```python
from build123d import *

# Parameters (mm, degrees)
SKETCH1_W                                         = 19.05
SKETCH1_H                                         = 19.05
BOSS_EXTRUDE1_DEPTH                               = 6.35
SKETCH2_W                                         = 6.444113488
SKETCH2_H                                         = 19.05
BOSS_EXTRUDE2_DEPTH                               = 12.7
CSK_FOR_8_FLAT_HEAD_MACHINE_SCREW_100_D           = 4.9149
CSK_FOR_8_FLAT_HEAD_MACHINE_SCREW_100_DEPTH       = 23.368
CSK_FOR_8_FLAT_HEAD_MACHINE_SCREW_100_CSINK_D     = 8.4328
CSK_FOR_8_FLAT_HEAD_MACHINE_SCREW_100_CSINK_ANGLE = 100
CSK_FOR_8_FLAT_HEAD_MACHINE_SCREW_100_TIP         = 1.476584928
SKETCH5_R                                         = 1.5875
CUT_EXTRUDE1_DEPTH                                = 12.7
FILLET1_R                                         = 2.54
FILLET2_R                                         = 7.62


with BuildPart() as part:
    # Sketch1 → Boss-Extrude1 (new body)
    with BuildSketch(Plane(origin=(0, 0, 0), x_dir=(1, 0, 0), z_dir=(0, 1, 0))):
        with Locations((9.525, 9.525)):
            Rectangle(SKETCH1_W, SKETCH1_H)
    extrude(amount=BOSS_EXTRUDE1_DEPTH)

    # Sketch2 → Boss-Extrude2 (add)
    with BuildSketch(Plane(origin=(0, 6.35, 0), x_dir=(1, 0, 0), z_dir=(0, 1, 0))):
        with Locations((3.222056744, 9.525)):
            Rectangle(SKETCH2_W, SKETCH2_H)
    extrude(amount=BOSS_EXTRUDE2_DEPTH)

    # CSK for #8 Flat Head Machine Screw (100)1
    with Locations(Plane(origin=(0, 6.35, 0), x_dir=(1, 0, 0), z_dir=(0, 1, 0))):
        with Locations((12.7, 13.97), (12.7, 5.08)):
            CounterSinkHole(CSK_FOR_8_FLAT_HEAD_MACHINE_SCREW_100_D / 2, CSK_FOR_8_FLAT_HEAD_MACHINE_SCREW_100_CSINK_D / 2, depth=CSK_FOR_8_FLAT_HEAD_MACHINE_SCREW_100_DEPTH, counter_sink_angle=CSK_FOR_8_FLAT_HEAD_MACHINE_SCREW_100_CSINK_ANGLE)
            with Locations((0, 0, -(CSK_FOR_8_FLAT_HEAD_MACHINE_SCREW_100_DEPTH + CSK_FOR_8_FLAT_HEAD_MACHINE_SCREW_100_TIP / 2))):  # 118° drill point
                Cone(0, CSK_FOR_8_FLAT_HEAD_MACHINE_SCREW_100_D / 2, CSK_FOR_8_FLAT_HEAD_MACHINE_SCREW_100_TIP, mode=Mode.SUBTRACT)

    # Sketch5 → Cut-Extrude1 (cut)
    with BuildSketch(Plane(origin=(6.444113488, 0, 0), x_dir=(0, 0, -1), z_dir=(1, 0, 0))):
        with Locations((9.525, 12.7)):
            Circle(SKETCH5_R)
    extrude(amount=-CUT_EXTRUDE1_DEPTH, mode=Mode.SUBTRACT)

    # Fillet1
    fillet1_edges = [part.edges().sort_by_distance(p)[0] for p in [
        (6.444113488, 6.35, -9.525),
    ]]
    fillet(fillet1_edges, radius=FILLET1_R)

    # Fillet2
    fillet2_edges = [part.edges().sort_by_distance(p)[0] for p in [
        (0, 0, -9.525),
    ]]
    fillet(fillet2_edges, radius=FILLET2_R)


solid = part.part
```
The model under review builds one solid part; all positions refer to its coordinate system, in mm. A direction names the side the tool comes from. Round coordinates to 2 decimals unless told otherwise and drop trailing zeros. Order: outer loops, then holes, each group sorted by start corner. A loop starts at its lowest first (then second) coordinate and runs counter-clockwise, first axis right, second up. Notation, with made-up numbers: (56, -10.5) -> (67, -10.5) arc R22 ccw to (67, 5.5) -> close; hole circle Ø8 at (36, 27). An arc over 180 degrees is marked (long way). One line per item, written item: value. Start each with the question number.
Q1. Take a section at B-B (x = 12.7). Write out the cut boundary in (y, z).
Q2. Take a section at D-D (y = 17.5). Write out the cut boundary in (x, z).
Q3. Mouldability with a two-part tool opening along Z and no side actions: class faces 3 (the face through (19.05, 3, -9)), 4 (the face through (14.65, 2.403, -3.585)), 5 (the face through (5, 7, -19.05)) as released by +Z, released by -Z, zero draft, split by the parting line, or undercut.
Q4. Wall thickness on line 1 (Z direction, x = 12.7, y = 3.55); line 2 (Y direction, x = 13, z = -9.5); line 3 (X direction, y = 16, z = -14.5): over which ranges is each line inside the solid? List them lowest first.
Q5. Machinability: for faces 1 (the face through (13, 0, -10)), 2 (the face through (6.444, 15, -9)), which of the approach directions +Z, -Z, +X, -X, +Y, -Y give a long, thin tool a straight path to every point of the face, cutting with its end or side? Answer none if there is none.
Q6. Take a section at A-A (y = 12.7). Write out the cut boundary in (x, z).
Q7. Clearance check with flat-ended pins moving along their axes: pin 1 Ø1.5 at (y, z) = (13, -3) entering from +X; pin 2 Ø5 at (x, z) = (13.5, -7) entering from +Y. State where each tip first meets the part, or that it passes through.
Reported:
1. outline: (0, -19.05) -> (6.35, -19.05) -> (6.35, -18.19) -> (4.87, -16.43) -> (0, -16.43) -> close; (0, -11.51) -> (4.87, -11.51) -> (6.35, -9.75) -> (6.35, -9.3) -> (4.87, -7.54) -> (0, -7.54) -> close; (0, -2.62) -> (4.87, -2.62) -> (6.35, -0.86) -> (6.35, 0) -> (0, 0) -> close
2. outline: (0, -19.05) -> (6.44, -19.05) -> (6.44, 0) -> (0, 0) -> close
3. face 3: zero draft
3. face 4: undercut
3. face 5: released by -Z
4. line 1: z = -19.05 to -16.43, -11.51 to -7.54, -2.62 to 0
4. line 2: y = 0 to 6.35
4. line 3: x = 0 to 6.44
5. face 1: +Z, -Z, +X, -X, -Y
5. face 2: +Z, -Z, +X, +Y
6. outline: (0, -19.05) -> (6.44, -19.05) -> (6.44, -11.11) -> (0, -11.11) -> close; (0, -7.94) -> (6.44, -7.94) -> (6.44, 0) -> (0, 0) -> close
7. pin 1: stops at x = 6.44
7. pin 2: stops at y = 6.35
